Part model, mm, in its own coordinate system. Give positions to 0.01 mm unless a question says otherwise; leave off trailing zeros. Order: outer loops, then holes, each group sorted by start corner. A loop starts at its lowest first (then second) coordinate and runs counter-clockwise, first axis right, second up. Notation, with made-up numbers: (59.25, -15) -> (109.25, -15) arc R11 cw to (109.25, 4) -> close; hole circle Ø2 at (-33, 3). An arc over 180 degrees is marked (long way). Write item = value, one per line. Start each with the question number.
Item 1: Band-saw the part on D-D on z = 15.09. Write the cut outline in (x, y) (3 decimals), plus the area to 3 significant figures.
Item 2: Band-saw the part on B-B on y = 0. Write the cut outline in (x, z) (3 decimals), plus the area to 3 significant figures.
Item 3: Pull direction Y, two halves, no side cores. Call faces 1 (the face through (12.34, 3.89, 15.03)), 2 (the face through (9, 10, 10.59)), 3 (the face through (10.333, -1.863, 14.121)): +Y half, -Y half, draft (parallel to the pull), parting line (faces both ways), or undercut.
Item 4: Drill centre lines: line 1 along Y through (x, z) = (0, 11) (3 decimals); line 2 along Z through (x, y) = (10, 0); line 3 along Z through (x, y) = (-15.5, 11.5). Where is each one in solid material? Low to high.
Item 5: Band-saw the part on C-C on y = -6. Write the cut outline in (x, z), plus the area to 3 significant figures.
Item 6: Band-saw the part on A-A on x = 0. Write the cut outline in (y, z) (3 decimals), plus the area to 3 significant figures.
Item 7: Flat gauge pins, fed straight in: P1, Ø4, axis at y = 4, z = 13, coming from the -X side; P2, Ø4, axis at y = -5, z = 7.5, coming from the -X side; P3, Ø5, axis at y = 6, z = 5.5, coming from the -X side. Where does each tip first touch, or does it go through?
```python
from build123d import *

# Parameters (mm, degrees)
SKETCH1_R               = 20.87
BOSS_EXTRUDE1_DEPTH     = 10.59
SKETCH2_R               = 12.94
BOSS_EXTRUDE2_DEPTH     = 9
CUT_EXTRUDE1_DEPTH      = 36.424312273
CUT_EXTRUDE1_DEPTH_BACK = 36.424312273
SKETCH3_R               = 8.075
CUT_EXTRUDE2_DEPTH      = 36.424312273
CUT_EXTRUDE2_DEPTH_BACK = 36.424312273
SKETCH4_R               = 2.1


with BuildPart() as part:
    # Sketch1 → Boss-Extrude1 (new body)
    with BuildSketch(Plane(origin=(0, 0, 0), x_dir=(0, 1, 0), z_dir=(0, 0, 1))):
        with Locations(Location((0, 0, 0), (0, 0, 270))):
            Circle(SKETCH1_R)
    extrude(amount=BOSS_EXTRUDE1_DEPTH)

    # Sketch2 → Boss-Extrude2 (add)
    with BuildSketch(Plane.XY.offset(10.59)):
        Circle(SKETCH2_R)
    extrude(amount=BOSS_EXTRUDE2_DEPTH)

    # Sketch3 → Cut-Extrude1 (cut, two sides: drawn at the far end of the back side and taken through both)
    with BuildSketch(Plane.XY.offset(19.59).offset(-CUT_EXTRUDE1_DEPTH_BACK)):
        Circle(SKETCH3_R)
    extrude(amount=CUT_EXTRUDE1_DEPTH + CUT_EXTRUDE1_DEPTH_BACK, mode=Mode.SUBTRACT)

    # Sketch4 → Cut-Extrude2 (cut, two sides: drawn at the far end of the back side and taken through both)
    with BuildSketch(Plane.YZ.offset(-CUT_EXTRUDE2_DEPTH_BACK)):
        with Locations(Location((0, 15.09, 0), (0, 0, 270))):
            Circle(SKETCH4_R)
    extrude(amount=CUT_EXTRUDE2_DEPTH + CUT_EXTRUDE2_DEPTH_BACK, mode=Mode.SUBTRACT)


solid = part.part
```
Values found:
q1.outline = (-12.768, -2.1) arc R12.94 ccw to (12.768, -2.1) -> (7.797, -2.1) arc R8.075 cw to (-7.797, -2.1) -> close; (-12.768, 2.1) -> (-7.797, 2.1) arc R8.075 cw to (7.797, 2.1) -> (12.768, 2.1) arc R12.94 ccw to start
q1.area = 280 mm^2
q2.outline = (-20.87, 0) -> (-8.075, 0) -> (-8.075, 12.99) -> (-12.94, 12.99) -> (-12.94, 10.59) -> (-20.87, 10.59) -> close; (-12.94, 17.19) -> (-8.075, 17.19) -> (-8.075, 19.59) -> (-12.94, 19.59) -> close; (8.075, 0) -> (20.87, 0) -> (20.87, 10.59) -> (12.94, 10.59) -> (12.94, 12.99) -> (8.075, 12.99) -> close; (8.075, 17.19) -> (12.94, 17.19) -> (12.94, 19.59) -> (8.075, 19.59) -> close
q2.area = 318 mm^2
q3.face_1 = parting line
q3.face_2 = draft
q3.face_3 = undercut
q4.line_1 = -12.94 to -8.075, 8.075 to 12.94
q4.line_2 = 0 to 12.99, 17.19 to 19.59
q4.line_3 = 0 to 10.59
q5.outline = (-19.99, 0) -> (-5.4, 0) -> (-5.4, 19.59) -> (-11.46, 19.59) -> (-11.46, 10.59) -> (-19.99, 10.59) -> close; (5.4, 0) -> (19.99, 0) -> (19.99, 10.59) -> (11.46, 10.59) -> (11.46, 19.59) -> (5.4, 19.59) -> close
q5.area = 418 mm^2
q6.outline = (-20.87, 0) -> (-8.075, 0) -> (-8.075, 19.59) -> (-12.94, 19.59) -> (-12.94, 10.59) -> (-20.87, 10.59) -> close; (8.075, 0) -> (20.87, 0) -> (20.87, 10.59) -> (12.94, 10.59) -> (12.94, 19.59) -> (8.075, 19.59) -> close
q6.area = 359 mm^2
q7.P1 = -12.78
q7.P2 = -20.65
q7.P3 = -20.57
